Could you check a few things on this drawing? It's one solid part, dimensions in mm from its lowest x, y, z. A direction names the side the tool comes from. Give positions to 0.01 mm unless a question says otherwise; leave off trailing zeros. Order: outer loops, then holes, each group sorted by start corner. A loop starts at its lowest first (then second) coordinate and runs counter-clockwise, first axis right, second up.
Item 1: I want a section at A-A, the plane y = 5. Write out the boundary of the cut face in (x, z).
Item 2: If I drill on line 1 along X through (y, z) = (15.5, 52); line 2 along Z through (x, y) = (128, 37.5); line 3 along Y through (x, z) = (37, 9), over which ranges is the centre line in solid material (lowest first)?
Item 3: I want a section at C-C, the plane y = 25. Write out the boundary of the cut face in (x, z), then the cut area to 3 significant figures.
Item 4: I want a section at D-D, the plane x = 107. Write out the boundary of the cut face in (y, z).
Item 5: Which directions (+Z, -Z, +X, -X, +Y, -Y) give clear straight access to the entire face, cutting with the end or side of a thin tool? Please do the marked faces 5 and 6.
Item 6: I want a section at B-B, the plane z = 44.5. Write out the boundary of the cut face in (x, y).
Item 7: If we mould it in two halves opening along X, with no side actions, what happens to the marked faces 1, 2, 3 and 4? For each: +X half, -X half, draft (parallel to the pull), parting line (faces both ways), or undercut.
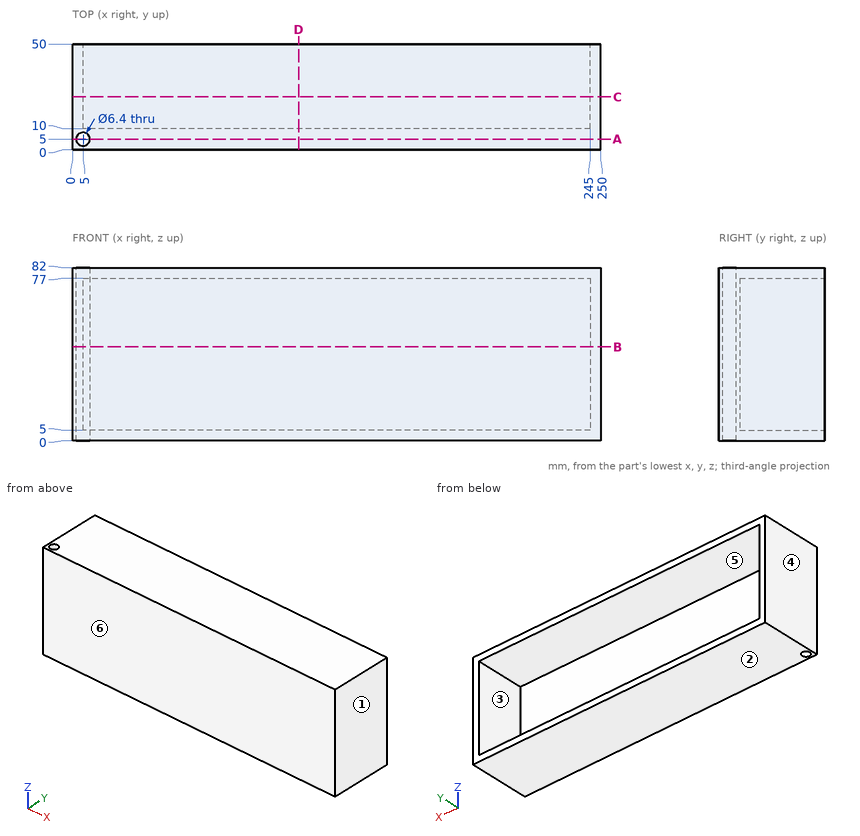
Results list:
1. outline: (0, 0) - (1.8, 0) - (1.8, 82) - (0, 82) - close; (8.2, 0) - (250, 0) - (250, 82) - (8.2, 82) - close
2. line 1: x = 0 to 5, 245 to 250
2. line 2: z = 0 to 5, 77 to 82
2. line 3: y = 0 to 10
3. outline: (0, 0) - (250, 0) - (250, 82) - (0, 82) - close; hole (5, 5) - (245, 5) - (245, 77) - (5, 77) - close
3. area: 3,220 mm2
4. outline: (0, 0) - (50, 0) - (50, 5) - (10, 5) - (10, 77) - (50, 77) - (50, 82) - (0, 82) - close
5. face 5: +Y
5. face 6: +Z, -Z, +X, -X, -Y
6. outline: (0, 0) - (250, 0) - (250, 50) - (245, 50) - (245, 10) - (5, 10) - (5, 50) - (0, 50) - close; hole circle Ø6.4 at (5, 5)
7. face 1: +X half
7. face 2: draft
7. face 3: undercut
7. face 4: -X half
